```python
from build123d import *

# Parameters (mm, degrees)
F0_R     = 5
F0_R_2   = 4
F0_R_3   = 0.2
F1_DEPTH = 1
F2_DEPTH = 0.5
F4_DEPTH = 25
F5_SIZE2 = 0.288665
F5_SIZE  = 0.49999


# Not quite as in the source:
# - a fillet or chamfer is up to 0.001 mm smaller than in the source, because OpenCascade refuses the exact size


with BuildPart() as f1:
    # F0 (on Top) → F1 (new body)
    with BuildSketch(Plane.XY):
        Circle(F0_R)
        Circle(F0_R_2, mode=Mode.SUBTRACT)
        with Locations((4.65, 0)):
            Circle(F0_R_3, mode=Mode.SUBTRACT)
    extrude(amount=F1_DEPTH)

    # F0 (on Top) → F2 (join)
    with BuildSketch(Plane.XY):
        Circle(F0_R_2)
    extrude(amount=F2_DEPTH)

    # F3 (on face) → F4 (cut)
    with BuildSketch(Plane.XY.offset(0.5)):
        with BuildLine():
            ThreePointArc((0.4898979486, -0.1), (0.4974680765, -0.050254481), (0.5, 0))
            ThreePointArc((0.5, 0), (0.4974680765, 0.050254481), (0.4898979486, 0.1))
            ThreePointArc((0.4898979486, 0.1), (-0.5, 0), (0.4898979486, -0.1))
        make_face()
        with BuildLine():
            ThreePointArc((0.4898979486, 0.1), (0.4974680765, 0.050254481), (0.5, 0))
            ThreePointArc((0.5, 0), (0.4974680765, -0.050254481), (0.4898979486, -0.1))
            Line((0.4898979486, -0.1), (0.6898979486, -0.1))
            Line((0.6898979486, -0.1), (0.6898979486, 0))
            Line((0.6898979486, 0), (0.6898979486, 0.1))
            Line((0.6898979486, 0.1), (0.4898979486, 0.1))
        make_face()
    extrude(amount=-F4_DEPTH, mode=Mode.SUBTRACT)

    # F5 (size 0.5 and 0.2886751346 in the source; OpenCascade refuses exactly that, so slightly less here)
    f5_edges = [f1.edges().sort_by_distance(p)[0] for p in [
        (-4, 0, 1),
    ]]
    f5_side = f1.faces().sort_by_distance((-4, 0, 0.75))[0]
    chamfer(f5_edges, length=F5_SIZE, length2=F5_SIZE2, reference=f5_side)


solid = f1.part
```
Verification items for the finished model (mm, model axes). Round coordinates to 2 decimals unless told otherwise and drop trailing zeros. Order: outer loops, then holes, each group sorted by start corner. A loop starts at its lowest first (then second) coordinate and runs counter-clockwise, first axis right, second up. Notation, with made-up numbers: (-8, 29) - (10, 29) arc R19 cw to (10, 61) - close; hole circle Ø8 at (59, 66). An arc over 180 degrees is marked (long way). Use CSV: the item, a comma, the result in double quotes. Start each with the question number.
1) Section check C-C, the plane x = 4.65. Record the cut outline in (y, z).
2) Mould release check, pull along X, two halves, no side actions. Record for faces 1 (the flat face through (1, 0, 0)), 2 (the cylindrical face through (-1.08, -4.88, 0.49)), 3 (the flat face through (1, 0, 0.5)): +X half, -X half, draft (parallel to the pull), parting line (faces both ways), or undercut.
3) Go/stop test with flat-tipped pins: P1, Ø3, axis at x = -2.5, y = -0.5, coming from the +Z side; P2, Ø1, axis at x = -1.5, y = -1, coming from the +Z side. Record where each tip stops, or that it passes through.
4) Section check B-B, the plane z = 0.15. Record the cut outline in (x, y), plus the area to 3 significant figures.
5) Thickness scan on L1, parallel to Y at x = 0, z = 0.3; L2, parallel to Z at x = 2.75, y = 1.5; L3, parallel to X at y = -3, z = 0.2. Record the ranges inside material, lowest first.
Answers:
1,outline,"(-1.84, 0) - (-0.2, 0) - (-0.2, 1) - (-1.84, 1) - close; (0.2, 0) - (1.84, 0) - (1.84, 1) - (0.2, 1) - close"
2,face 1,"draft"
2,face 2,"parting line"
2,face 3,"undercut"
3,P1,"stops at z = 0.59"
3,P2,"stops at z = 0.5"
4,outline,"circle Ø10 at (0, 0); hole (0.49, -0.1) - (0.69, -0.1) - (0.69, 0.1) - (0.49, 0.1) arc R0.5 ccw (long way) to start; hole circle Ø0.4 at (4.65, 0)"
4,area,"77.6 mm²"
5,L1,"y = -5 to -0.5, 0.5 to 5"
5,L2,"z = 0 to 0.5"
5,L3,"x = -4 to 4"
